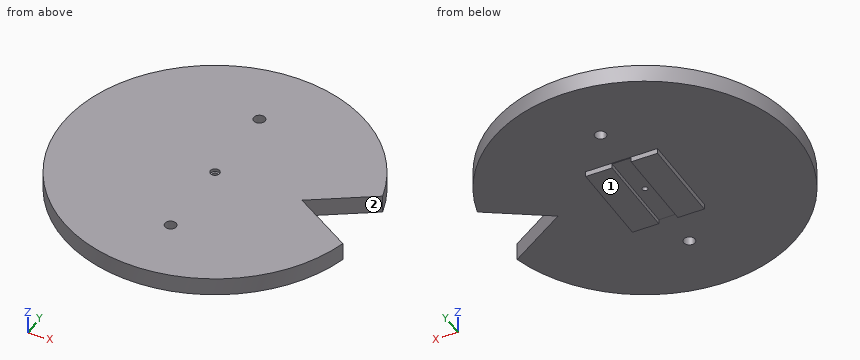
Autodesk Inventor part; units mm, degrees
ref_plane "Work Plane1" through (0, 15, 0) normal (0, 1, 0) x (-1, 0, 0)
ref_plane "Work Plane2" through (0, -15, 0) normal (0, 1, 0) x (-1, 0, 0)
ref_plane "YZ Plane" through (0, 0, 0) normal (1, 0, 0) x (0, 1, 0)
sketch "Sketch1" plane through (0, 0, 0) normal (0, 0, 1) x (1, 0, 0)
  circle A0 centre (0, 0) radius 85
  line L0 (0, -85) -> (0, 85)
  line L1 (-85, 0) -> (85, 0)
  circle A1 centre (0, -47.5) radius 3.175
  circle A2 centre (0, 47.5) radius 3.175
  line L2 (82.2887, 21.2973) -> (48.4298, 0)
  line L3 (48.4298, 0) -> (82.2887, -21.2973)
  dimension "d0" = 170
  dimension "d21" = 6.35
  dimension "d22" = 47.5
  dimension "d49" = 40
  dimension "d50" = 40
  dimension "d51" = 32.17
extrude "Extrusion1" add sketch "Sketch1" along normal blind 10
sketch "Sketch2" plane through (0, 0, 0) normal (0, 0, -1) x (-1, 0, 0)
  line L0 (-20, -25) -> (20, -25)
  line L1 (20, -25) -> (20, 25)
  line L2 (20, 25) -> (-20, 25)
  line L3 (-20, 25) -> (-20, -25)
  line L4 (0, -25) -> (0, 25)
  line L5 (5.3, -25) -> (5.3, 25)
  line L6 (-5.3, -25) -> (-5.3, 25)
  circle A0 centre (0, 0) radius 1.5
  point P0 (-5.3, -25)
  point P1 (5.3, -25)
  dimension "d3" = 40
  dimension "d4" = 50
  dimension "d18" = 3
  dimension "d25" = 5.3
  dimension "d27" = 10.6
extrude "Extrusion2" add sketch "Sketch2" along normal blind 3 contours L3 L2 L6 L0 | L5 L2 L1 L0
extrude "Extrusion3" add sketch "Sketch2" along normal blind 0.5 contours L6 L2 L4 A0 L0 | L4 A0 L2 L5 L0 | A0 L4 | L4 A0
extrude "Extrusion4" cut sketch "Sketch2" along normal through all both and the other way through all contours A0 L4 | L4 A0
extrude "Extrusion5" cut sketch "Sketch1" along normal through all contours A2 L0 | L0 A2 | A1 L0 | L0 A1
thread "Thread1"
sketch "Sketch3" plane through (0, 0, 10) normal (0, 0, 1) x (1, 0, 0)
  circle A0 centre (0, 0) radius 2.6
  dimension "d30" = 5.2
extrude "Extrusion6" cut sketch "Sketch3" against normal blind 1.7
ref_plane "Work Plane1" through (0, 15, 0) normal (0, 1, 0) x (-1, 0, 0)
ref_plane "Work Plane2" through (0, -15, 0) normal (0, 1, 0) x (-1, 0, 0)
extrude "Extrusion9" cut sketch "Sketch1" along normal blind 10 contours L1 L2 A0 | A0 L3 L1
properties part number "Base" material "Wood (Maple)"
Model file for the job. Use its own axes, mm. Face numbers are marked on the shaded views. A direction names the side the tool comes from. Give positions to 0.01 mm unless a question says otherwise; leave off trailing zeros. Loops run counter-clockwise (first coordinate to the right, second up) from the corner with the lowest first, then second, coordinate; pieces in that order, holes last. Notation, with made-up numbers: (69, 26.5) - (106, 26.5) arc R18 ccw to (106, 44.5) - close; hole circle Ø7 at (46, -16.5). An arc over 180 degrees is marked (long way). One line per item, written item: value. Start each with the question number.
1. Which spindle directions (+Z, -Z, +X, -X, +Y, -Y) get a long thin tool onto all of the face, cutting with end or side? Do the marked faces 1 and 2. Say none if no direction does.
2. Slice it at B-B (x = 53.5). List the corners of the cut face in (y, z).
3. Slice it at C-C (z = 5.25). List the corners of the cut face in (x, y) (3 decimals).
4. Probe L1, parallel to Y at x = 0, z = 5 (3 decimals); L2, parallel to Z at x = -9.5, y = -27; L3, parallel to X at y = 47.5, z = 1.75 (3 decimals). List the from-to ranges inside material, lowest first. Write a range as from..to.
5. Pin check, flat tips, straight feed: pin 1 (6 mm diameter, centred on x = 5.5, z = 7, fed in from +Y); pin 2 (5 mm diameter, centred on x = 57, z = 2.5, fed in from -Y); pin 3 (3.5 mm diameter, centred on x = -10, z = -1, fed in from -Y). Stop position of each tip, or through.
6. Slice it at D-D (y = 32.5). List the corners of the cut face in (x, z), plus the area to 3 significant figures.
7. Slice it at A-A (y = -47.5). List the corners of the cut face in (x, z) (3 decimals), plus the area to 3 significant figures.
Solution:
1. face 1: -Z, +X, -X, +Y, -Y
1. face 2: +Z, -Z, +X
2. outline: (-66.05, 0) - (-3.19, 0) - (-3.19, 10) - (-66.05, 10) - close; (3.19, 0) - (66.05, 0) - (66.05, 10) - (3.19, 10) - close
3. outline: (48.43, 0) - (82.289, 21.297) arc R85 ccw (long way) to (82.289, -21.297) - close; hole circle Ø6.35 at (0, -47.5); hole circle Ø6.35 at (0, 47.5); hole circle Ø3 at (0, 0)
4. L1: y = -85..-50.675, -44.325..-1.5, 1.5..44.325, 50.675..85
4. L2: z = 0..10
4. L3: x = -70.489..-3.175, 3.175..70.489
5. pin 1: stops at y = 84.96
5. pin 2: stops at y = -65.23
5. pin 3: stops at y = -84.57
6. outline: (-78.54, 0) - (78.54, 0) - (78.54, 10) - (-78.54, 10) - close
6. area: 1,570 mm^2
7. outline: (-70.489, 0) - (-3.175, 0) - (-3.175, 10) - (-70.489, 10) - close; (3.175, 0) - (70.489, 0) - (70.489, 10) - (3.175, 10) - close
7. area: 1,350 mm^2
